Source: CAD feature listing. Evaluate the final solid. Frame: model axes, mm. Face numbers are marked on the shaded views. Give positions to 0.01 mm unless a question says otherwise; leave off trailing zeros. Loops run counter-clockwise (first coordinate to the right, second up) from the corner with the lowest first, then second, coordinate; pieces in that order, holes last. Notation, with made-up numbers: (1.25, -25.5) - (33.25, -25.5) arc R23 cw to (33.25, 3.5) - close; hole circle Ø6 at (12.25, -38.75). An arc over 180 degrees is marked (long way). Write each question's results on one line, items separated by ' | '. Start each with the question number.
(1) Cut plane C-C on z = 6.5. Return the cut outline in (x, y), then the cut area to 3 significant figures.
(2) Material intervals for line 1 along Y through (x, z) = (0, 14.25); line 2 along Y through (x, z) = (1.8, 5.5); line 3 along Y through (x, z) = (1.2, 4), sorted ascending. Write a range as [from, to].
(3) Contact query for a flat-ended pin moving along its axis: pin 1 (1.5 mm diameter, centred on x = -1, z = 16, fed in from +Y). Output: stop coordinate, or through.
(4) Pull-direction query (Y, two-part tool) for the marked faces 1 and 2; classes: pulls with the +Y half, pulls with the -Y half, needs draft (parallel to the pull), parting line crosses it, or undercut.
(5) Cut plane D-D on y = 2. Return the cut outline in (x, z), then the cut area to 3 significant figures.
(6) Cut plane A-A on x = 0. Return the cut outline in (y, z).
from build123d import *

# Parameters (mm, degrees)
F0_R     = 2.75
F1_DEPTH = 2
F2_R     = 2.75
F2_R_2   = 0.5
F3_DEPTH = 16
F4_R     = 2.75
F5_DEPTH = 2


with BuildPart() as f1:
    # F0 (on Top) → F1 (new body)
    with BuildSketch(Plane.XY):
        Circle(F0_R)
    extrude(amount=F1_DEPTH)

    # F2 (on face) → F3 (join)
    with BuildSketch(Plane.XY.offset(2)):
        Circle(F2_R)
        Circle(F2_R_2, mode=Mode.SUBTRACT)
    extrude(amount=F3_DEPTH)

    # F4 (on face) → F5 (join)
    with BuildSketch(Plane.XY.offset(18)):
        Circle(F4_R)
    extrude(amount=F5_DEPTH)


solid = f1.part
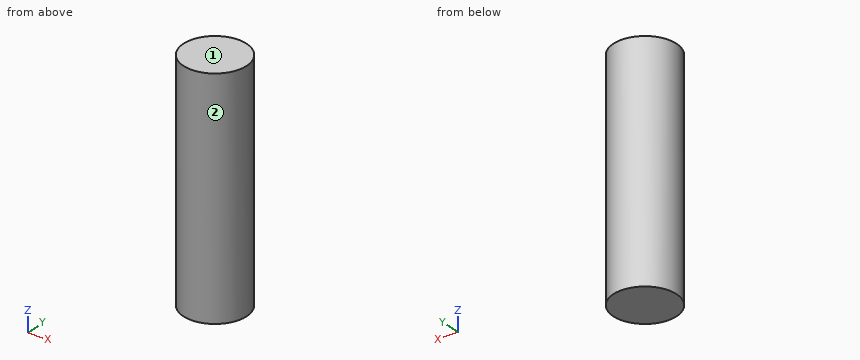
Ans:
1) outline: circle Ø5.5 at (0, 0); hole circle Ø1 at (0, 0) | area: 23.0 mm^2
2) line 1: [-2.75, -0.5], [0.5, 2.75] | line 2: [-2.08, 2.08] | line 3: [-2.47, 2.47]
3) pin 1: y = 2.74
4) face 1: needs draft | face 2: parting line crosses it
5) outline: (-1.89, 0) - (1.89, 0) - (1.89, 20) - (-1.89, 20) - close | area: 75.5 mm^2
6) outline: (-2.75, 0) - (2.75, 0) - (2.75, 20) - (-2.75, 20) - close; hole (-0.5, 2) - (0.5, 2) - (0.5, 18) - (-0.5, 18) - close
